Read the model definition and answer for the solid it produces. Units are mm, in the model's axes. Face numbers are marked on the shaded views. A direction names the side the tool comes from. Coordinates: 2 decimals unless noted, no trailing zeros. Order: outer loops, then holes, each group sorted by start corner. A loop starts at its lowest first (then second) coordinate and runs counter-clockwise, first axis right, second up. Notation, with made-up numbers: M 61.25,77.25 L 102.25,77.25 A18 ccw 102.25,94.25 Z; hole C -20.75,79.25 d2. An arc over 180 degrees is marked long. Write each question's results on one line, items separated by ' | '.
```python
from build123d import *

# Parameters (mm, degrees)
SKETCH1_W           = 6
SKETCH1_H           = 4
BOSS_EXTRUDE1_DEPTH = 3
BOSS_EXTRUDE2_DEPTH = 2


with BuildPart() as part:
    # Sketch1 → Boss-Extrude1 (new body)
    with BuildSketch(Plane(origin=(0, 0, 0), x_dir=(1, 0, 0), z_dir=(0, 1, 0))):
        with Locations((3, 2)):
            Rectangle(SKETCH1_W, SKETCH1_H)
    extrude(amount=BOSS_EXTRUDE1_DEPTH)

    # Sketch3 → Boss-Extrude2 (add)
    with BuildSketch(Plane(origin=(0, 3, 0), x_dir=(1, 0, 0), z_dir=(0, 1, 0))):
        Polygon((6, 4), (6, 0), (4.997854063, 0), (2, 4), align=None)
    extrude(amount=BOSS_EXTRUDE2_DEPTH)


solid = part.part
```
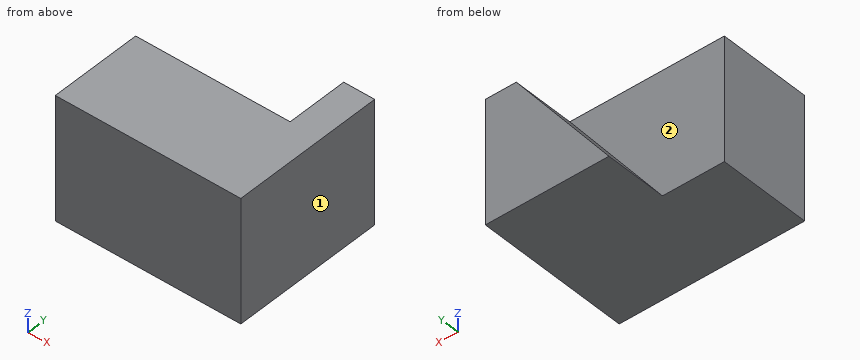
(1) The part is cut by section D-D, the plane x = 0.55. Write down the section's boundary in (y, z), then the cut area to 3 significant figures.
Conclusion:
outline: M 0,-4 L 3,-4 L 3,0 L 0,0 Z | area: 12.0 mm²
(2) For the marked faces 1 and 2, determine the directions among +Z, -Z, +X, -X, +Y, -Y from which every point of the face is accessible in a straight line to the end or side of a thin tool.
Conclusion:
face 1: +Z, -Z, +X, +Y, -Y | face 2: +Z, -X, +Y
(3) The part is cut by section A-A, the plane z = -1.8. Write down the section's boundary in (x, y), then the cut area to 3 significant figures.
Conclusion:
outline: M 0,0 L 6,0 L 6,5 L 3.65,5 L 3.65,3 L 0,3 Z | area: 22.7 mm²
(4) The part is cut by section B-B, the plane x = 2.2. Write down the section's boundary in (y, z).
Conclusion:
outline: M 0,-4 L 5,-4 L 5,-3.73 L 3,-3.73 L 3,0 L 0,0 Z
(5) The part is cut by section C-C, the plane y = 4.4. Write down the section's boundary in (x, z).
Conclusion:
outline: M 2,-4 L 6,-4 L 6,0 L 5,0 Z
(6) Straight lines are drawn through the part: line 1 (Y direction, x = 2.25, z = -1.65); line 2 (X direction, y = 4.1, z = -2.75); line 3 (X direction, y = 3.4, z = -1.2). For each, find the intervals that lie inside material, in ascending order.
Conclusion:
line 1: 0 to 3 | line 2: 2.94 to 6 | line 3: 4.1 to 6
